The model under review builds one solid part; all positions refer to its coordinate system, in mm. A direction names the side the tool comes from. Round coordinates to 2 decimals unless told otherwise and drop trailing zeros. Write each loop counter-clockwise with the first axis right and the second up, starting at its lowest first coordinate (ties: lowest second). Pieces come first, ordered by that corner, then holes.
Item 1: Machinability: for faces 1 (the face through (-4.315, -0.054, 2.966)), 2 (the face through (0, 1.5, 3)), 3 (the face through (-2.226, -1.762, 2.966)), which of the approach directions +Z, -Z, +X, -X, +Y, -Y give a long, thin tool a straight path to every point of the face, cutting with its end or side? Answer none if there is none.
Item 2: Add section B-B (x = 0). Give the boundary of the cut face in (y, z), plus the area to 3 significant figures.
Item 3: Add section A-A (y = 0). Give the boundary of the cut face in (x, z).
Item 4: Clearance check with flat-ended pins moving along their axes: pin 1 Ø2 at (x, z) = (0, 4) entering from +Y; pin 2 Ø2 at (x, y) = (-1.5, -2.5) entering from +Z; pin 3 Ø1 at (x, z) = (0, 5) entering from -Y. State where each tip first meets the part, or that it passes through.
Item 5: To check wall thickness, follow L1, parallel to Y at x = -6.25, z = 2.6; L2, parallel to Y at x = 6.75, z = 4.8; L3, parallel to X at y = -2.75, z = 3.05. State the ranges of each line that lie inside material, in increasing order.
Item 6: Draft analysis for pull direction Y (two halves, no side actions). For faces 4 (the face through (4.42, 0.06, 2.97)), 5 (the face through (0, 0, 6)), 6 (the face through (2.282, 1.788, 2.966)), 7 (the face through (-5.572, -3.804, 2.966)), state which applies: +Y half, -Y half, draft (parallel to the pull), parting line (faces both ways), or undercut.
```python
from build123d import *

# Parameters (mm, degrees)
PAD_DEPTH    = 6
CHAMFER_SIZE = 0.6


with BuildPart() as part:
    # Sketch → Pad (new body)
    with BuildSketch(Plane.XY):
        with BuildLine():
            ThreePointArc((7.729552, 1.9), (9.097303, 2.259521), (8.737782, 3.627273))
            ThreePointArc((8.737782, 3.627273), (5.853481, 4.129368), (3.341874, 2.625))
            ThreePointArc((1, 1.5), (2.299038, 1.795837), (3.341874, 2.625))
            Line((1, 1.5), (-1, 1.5))
            ThreePointArc((-3.261843, 2.529197), (-2.242496, 1.769395), (-1, 1.5))
            ThreePointArc((-3.261843, 2.529197), (-5.535711, 3.798298), (-8.097261, 3.32973))
            ThreePointArc((-8.097261, 3.32973), (-8.460121, 1.96286), (-7.093251, 1.6))
            ThreePointArc((-7.093251, -1.6), (-4.314543, 0), (-7.093251, 1.6))
            ThreePointArc((-7.093251, -1.6), (-8.460121, -1.96286), (-8.097261, -3.32973))
            ThreePointArc((-8.097261, -3.32973), (-5.535711, -3.798298), (-3.261843, -2.529197))
            ThreePointArc((-1, -1.5), (-2.242496, -1.769395), (-3.261843, -2.529197))
            Line((1, -1.5), (-1, -1.5))
            ThreePointArc((3.341874, -2.625), (2.299038, -1.795837), (1, -1.5))
            ThreePointArc((3.341874, -2.625), (5.853481, -4.129368), (8.737782, -3.627273))
            ThreePointArc((8.737782, -3.627273), (9.097303, -2.259521), (7.729551, -1.9))
            ThreePointArc((7.729552, 1.9), (4.420498, 0), (7.729551, -1.9))
        make_face()
    extrude(amount=PAD_DEPTH)

    # Chamfer
    chamfer_edges = [part.edges().sort_by_distance(p)[0] for p in [
        (0, -1.5, 6),
        (0, -1.5, 0),
    ]]
    chamfer(chamfer_edges, length=CHAMFER_SIZE)


solid = part.part
```
Numbers:
1. face 1: +Z, -Z
1. face 2: +Z, -Z, +Y
1. face 3: +Z, -Z, -Y
2. outline: (-1.5, 0.6) - (-0.9, 0) - (0.9, 0) - (1.5, 0.6) - (1.5, 5.4) - (0.9, 6) - (-0.9, 6) - (-1.5, 5.4) - close
2. area: 17.3 mm2
3. outline: (-4.31, 0.6) - (-3.71, 0) - (3.82, 0) - (4.42, 0.6) - (4.42, 5.4) - (3.82, 6) - (-3.71, 6) - (-4.31, 5.4) - close
4. pin 1: stops at y = 1.5
4. pin 2: stops at z = 5.46
4. pin 3: stops at y = -1.5
5. L1: y = -3.85 to -1.85, 1.85 to 3.85
5. L2: y = -4.2 to -2.2, 2.2 to 4.2
5. L3: x = -8.55 to -3.47, 3.45 to 9.23
6. face 4: undercut
6. face 5: draft
6. face 6: +Y half
6. face 7: -Y half
